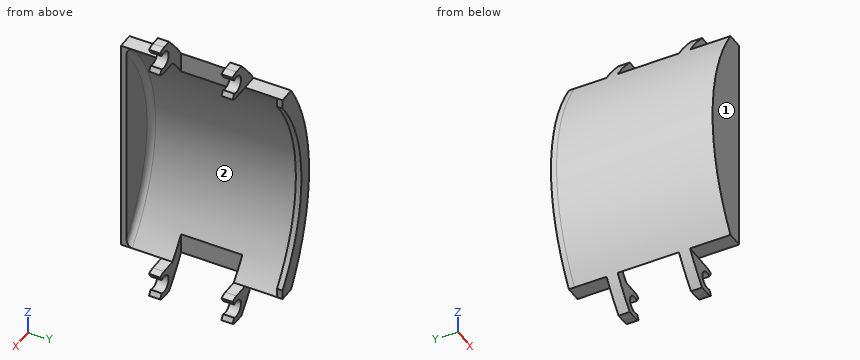
```python
from build123d import *

# Parameters (mm, degrees)
SKETCH2_R               = 3.048
BOSS_EXTRUDE1_DEPTH     = 56
CUT_EXTRUDE2_DEPTH      = 118.2998702
CUT_EXTRUDE3_DEPTH      = 117.054836818
CUT_EXTRUDE3_DEPTH_BACK = 117.054836818
SKETCH12_W              = 5.816526385
SKETCH12_H              = 22
SKETCH12_H_2            = 11.5
SKETCH12_H_3            = 14.5
SKETCH13_W              = 10.16
SKETCH13_H              = 11.5
SKETCH13_H_2            = 14.5
CUT_EXTRUDE4_DEPTH      = 10
FILLET1_R               = 10
BOSS_EXTRUDE2_DEPTH     = 2
FILLET2_R               = 2
BOSS_EXTRUDE3_DEPTH     = 2
SKETCH18_W              = 2.878327065
SKETCH18_H              = 3.541775271
SKETCH18_W_2            = 3.166541323
SKETCH18_H_2            = 3.584686202
CUT_EXTRUDE5_DEPTH      = 2
CUT_EXTRUDE7_DEPTH      = 109.465199714
CUT_EXTRUDE7_DEPTH_BACK = 109.465199714
SKETCH19_W              = 7.941935835
SKETCH19_H              = 22


with BuildPart() as part:
    # Sketch2 → Boss-Extrude1 (new body)
    with BuildSketch(Plane(origin=(0, 0, 0), x_dir=(1, 0, 0), z_dir=(0, 1, 0))):
        with BuildLine():
            Line((0.095782763, 91.44), (5.683782763, 91.44))
            ThreePointArc((5.683782763, 91.44), (10.763782763, 96.52), (5.683782763, 101.6))
            Line((5.683782763, 101.6), (2.421245281, 101.6))
            ThreePointArc((2.421245281, 101.6), (-17.340690554, 51.52), (2.421245281, 1.44))
            Line((2.421245281, 1.44), (5.683782763, 1.44))
            ThreePointArc((5.683782763, 1.44), (10.763782763, 6.52), (5.683782763, 11.6))
            Line((5.683782763, 11.6), (0.095782763, 11.6))
            ThreePointArc((0.095782763, 11.6), (-15.340690554, 51.52), (0.095782763, 91.44))
        make_face()
        with Locations(Location((5.683782763, 96.52, 0), (0, 0, 270))):
            Circle(SKETCH2_R, mode=Mode.SUBTRACT)
        with Locations(Location((5.683782763, 6.52, 0), (0, 0, 90))):
            Circle(SKETCH2_R, mode=Mode.SUBTRACT)
    extrude(amount=BOSS_EXTRUDE1_DEPTH)

    # Sketch6 → Cut-Extrude2 (cut, symmetric)
    with BuildSketch(Plane(origin=(0, 56, 0), x_dir=(1, 0, 0), z_dir=(0, 1, 0))):
        Polygon((5.683782763, 6.52), (11.45705153, 16.593499718), (11.45705153, -3.406500282), align=None)
    cut_extrude2 = extrude(amount=CUT_EXTRUDE2_DEPTH, both=True, mode=Mode.SUBTRACT)

    # Mirror1: Cut-Extrude2 across plane
    add(cut_extrude2.mirror(Plane.XY.offset(-51.52)), mode=Mode.SUBTRACT)

    # Sketch12 → Cut-Extrude3 (cut, two sides: drawn at the far end of the back side and taken through both)
    with BuildSketch(Plane.XY.offset(-1.44).offset(-CUT_EXTRUDE3_DEPTH_BACK)):
        with Locations((5.329508474, 29.5)):
            Rectangle(SKETCH12_W, SKETCH12_H)
        with Locations((5.329508474, 50.25)):
            Rectangle(SKETCH12_W, SKETCH12_H_2)
        with Locations((5.329508474, 7.25)):
            Rectangle(SKETCH12_W, SKETCH12_H_3)
    extrude(amount=CUT_EXTRUDE3_DEPTH + CUT_EXTRUDE3_DEPTH_BACK, mode=Mode.SUBTRACT)

    # Sketch13 → Cut-Extrude4 (cut)
    with BuildSketch(Plane(origin=(2.421245281, 0, 0), x_dir=(0, 0, -1), z_dir=(1, 0, 0))):
        with Locations((6.52, 50.25)):
            Rectangle(SKETCH13_W, SKETCH13_H)
        with Locations((6.52, 7.25)):
            Rectangle(SKETCH13_W, SKETCH13_H_2)
        with Locations((96.52, 50.25)):
            Rectangle(SKETCH13_W, SKETCH13_H)
        with Locations((96.52, 7.25)):
            Rectangle(SKETCH13_W, SKETCH13_H_2)
    extrude(amount=-CUT_EXTRUDE4_DEPTH, mode=Mode.SUBTRACT)

    # Fillet1
    # the kernel refuses this fillet: 10 mm, written as the material it takes off along each edge
    with BuildSketch(Plane(origin=(2.421245281, 18.5, -91.44), x_dir=(0, 0, -1), z_dir=(0, 1, 0)), Plane(origin=(2.421245281, 40.5, -11.6), x_dir=(0, 0, 1), z_dir=(0, -1, 0))) as fillet1_piece_1:
        with BuildLine():
            CenterArc((6.411043164, 10), FILLET1_R, 230.125785038, 39.874214962)
            Line((0, 2.325462519), (0, 0))
            Line((0, 0), (6.411043164, 0))
        make_face()
    extrude(amount=22, mode=Mode.SUBTRACT)

    # Sketch15 → Boss-Extrude2 (add)
    with BuildSketch(Plane(origin=(0, 0, 0), x_dir=(-1, 0, 0), z_dir=(0, -1, 0))):
        with BuildLine():
            Line((-0.095782763, 11.6), (-0.095782763, 91.44))
            ThreePointArc((-0.095782763, 91.44), (15.340690554, 51.52), (-0.095782763, 11.6))
        make_face()
    extrude(amount=-BOSS_EXTRUDE2_DEPTH)

    # Fillet2
    fillet2_edges = [part.edges().sort_by_distance(p)[0] for p in [
        (-15.340690554, 2, -51.52),
    ]]
    fillet(fillet2_edges, radius=FILLET2_R)

    # Sketch17 → Boss-Extrude3 (add)
    with BuildSketch(Plane(origin=(0, 56, 0), x_dir=(1, 0, 0), z_dir=(0, 1, 0))):
        with BuildLine():
            Line((2.889782763, 91.44), (-5.523575239, 91.44))
            ThreePointArc((-5.523575239, 91.44), (-17.340690554, 51.52), (-5.523575239, 11.6))
            Line((-5.523575239, 11.6), (2.889782763, 11.6))
            ThreePointArc((2.889782763, 11.6), (-12.340690554, 51.52), (2.889782763, 91.44))
        make_face()
    extrude(amount=BOSS_EXTRUDE3_DEPTH)

    # Sketch18 → Cut-Extrude5 (cut)
    with BuildSketch(Plane(origin=(0, 58, 0), x_dir=(1, 0, 0), z_dir=(0, 1, 0))):
        with Locations((1.534946295, 13.370887636)):
            Rectangle(SKETCH18_W, SKETCH18_H)
        with Locations((1.679053424, 89.647656899)):
            Rectangle(SKETCH18_W_2, SKETCH18_H_2)
    extrude(amount=-CUT_EXTRUDE5_DEPTH, mode=Mode.SUBTRACT)

    # Sketch19 → Cut-Extrude7 (cut, two sides: drawn at the far end of the back side and taken through both)
    with BuildSketch(Plane.XY.offset(-11.6).offset(-CUT_EXTRUDE7_DEPTH_BACK)):
        with Locations((-1.549722637, 29.5)):
            Rectangle(SKETCH19_W, SKETCH19_H)
    extrude(amount=CUT_EXTRUDE7_DEPTH + CUT_EXTRUDE7_DEPTH_BACK, mode=Mode.SUBTRACT)


solid = part.part
```
Could you check a few things on this model? Use its own coordinates, in mm. Face numbers are marked on the shaded views. Give positions to 0.01 mm unless a question says otherwise; leave off trailing zeros. Order: outer loops, then holes, each group sorted by start corner. A loop starts at its lowest first (then second) coordinate and runs counter-clockwise, first axis right, second up.
Q1. I'm going to push flat-ended pins straight in: P1, Ø8, axis at x = -4, z = -58, coming from the +Y side; P2, Ø8, axis at y = 49.5, z = -32.5, coming from the -X side; P3, Ø6, axis at y = 34, z = -49.5, coming from the +X side; P4, Ø5.5, axis at x = 5.68, z = -6.52, coming from the -Y side. Where does each tip first touch, or does it pass through?
Q2. Suppose I cut it at A-A, the plane x = 3.75. Count the separate pieces of the cut face and the enclosed holes in it, and give its area (3 significant figures).
Q3. Suppose I cut it at C-C, the plane y = 54. Write out the boundary of the cut face in (x, z).
Q4. Suppose I cut it at B-B, the plane z = -96.52. Write out the boundary of the cut face in (x, y), and give its area (3 significant figures).
Q5. We'd pull the mould along Z, two halves only. Please class the marked faces 1 and 2: +Z half, -Z half, draft (parallel to the pull), parting line (faces both ways), or undercut.
Q6. If I drill on line 1 along Y through (x, z) = (-13, -50); line 2 along Y through (x, z) = (1.25, -92); line 3 along Y through (x, z) = (-4, -35), over which ranges is the centre line in solid material (lowest first)?
Solution:
1. P1: stops at y = 2
1. P2: stops at x = -15.79
1. P3: stops at x = -15.13
1. P4: passes through
2. separate pieces: 8
2. enclosed holes: 0
2. area: 87.2 mm2
3. outline: (-5.52, -91.44) - (0.1, -91.44) arc R59.34 cw to (0.1, -11.6) - (-5.52, -11.6) arc R73.34 ccw to start
4. outline: (-1.91, 14.5) - (2.64, 14.5) - (2.64, 18.5) - (-1.91, 18.5) - close; (-1.91, 40.5) - (2.64, 40.5) - (2.64, 44.5) - (-1.91, 44.5) - close
4. area: 36.4 mm2
5. face 1: draft
5. face 2: undercut
6. line 1: y = 0 to 2, 56 to 58
6. line 2: y = 14.5 to 18.5, 40.5 to 44.5
6. line 3: y = 0 to 2
